```python
from build123d import *

# Parameters (mm, degrees)
SKETCH3_R           = 2.201333333
SKETCH3_R_2         = 1.693333333
BOSS_EXTRUDE1_DEPTH = 914.4
CUT_EXTRUDE1_START  = -1219.2
CUT_EXTRUDE1_DEPTH  = 1219.2


with BuildPart() as part:
    # Sketch3 → Boss-Extrude1 (new, symmetric)
    with BuildSketch(Plane.XY):
        with BuildLine():
            Line((-1.778, 0), (-1.778, 1.27))
            ThreePointArc((-1.778, 1.27), (-1.536070654, 2.494011801), (-0.846666667, 3.533942971))
            Line((-0.846666667, 3.533942971), (2.413267273, 6.793876912))
            ThreePointArc((2.413267273, 6.793876912), (2.578074335, 6.903997469), (2.772477518, 6.942666667))
            Line((2.772477518, 6.942666667), (3.048, 6.942666667))
            ThreePointArc((3.048, 6.942666667), (3.467078619, 6.769078619), (3.640666667, 6.35))
            Line((3.640666667, 6.35), (3.640666667, 4.301066667))
            ThreePointArc((3.640666667, 4.301066667), (3.948165494, 3.558698827), (4.690533333, 3.2512))
            Line((4.690533333, 3.2512), (5.300133333, 3.2512))
            ThreePointArc((5.300133333, 3.2512), (6.042501173, 3.558698827), (6.35, 4.301066667))
            Line((6.35, 4.301066667), (6.35, 10.583333333))
            ThreePointArc((6.35, 10.583333333), (5.730042687, 12.080042687), (4.233333333, 12.7))
            Line((4.233333333, 12.7), (-4.233333333, 12.7))
            ThreePointArc((-4.233333333, 12.7), (-5.730042687, 12.080042687), (-6.35, 10.583333333))
            Line((-6.35, 10.583333333), (-6.35, 0))
            Line((-6.35, 0), (-1.778, 0))
        make_face()
        with Locations(Location((-2.116666667, 8.466666667, 0), (0, 0, 180))):
            Circle(SKETCH3_R, mode=Mode.SUBTRACT)
        with Locations(Location((3.429, 9.906, 0), (0, 0, 180))):
            Circle(SKETCH3_R_2, mode=Mode.SUBTRACT)
    extrude(amount=BOSS_EXTRUDE1_DEPTH, both=True)

    # Mirror1: part across plane


with BuildPart() as part_1:
    add(part.part)
    add(part.part.mirror(Plane.ZX))

    # Sketch4 → Cut-Extrude1 (cut)
    with BuildSketch(Plane(origin=(0, 0, -914.4), x_dir=(-1, 0, 0), z_dir=(0, 0, -1)).offset(CUT_EXTRUDE1_START)):
        with BuildLine():
            Line((1.778, 1.27), (1.778, -1.27))
            ThreePointArc((1.778, -1.27), (1.536070654, -2.494011801), (0.846666667, -3.533942971))
            Line((0.846666667, -3.533942971), (-2.413267273, -6.793876912))
            ThreePointArc((-2.413267273, -6.793876912), (-2.578074335, -6.903997469), (-2.772477518, -6.942666667))
            Line((-2.772477518, -6.942666667), (-3.048, -6.942666667))
            ThreePointArc((-3.048, -6.942666667), (-3.467078619, -6.769078619), (-3.640666667, -6.35))
            Line((-3.640666667, -6.35), (-3.640666667, -4.301066667))
            ThreePointArc((-3.640666667, -4.301066667), (-3.948165494, -3.558698827), (-4.690533333, -3.2512))
            Line((-4.690533333, -3.2512), (-5.300133333, -3.2512))
            ThreePointArc((-5.300133333, -3.2512), (-6.042501173, -3.558698827), (-6.35, -4.301066667))
            Line((-6.35, -4.301066667), (-6.35, -10.583333333))
            ThreePointArc((-6.35, -10.583333333), (-5.730042687, -12.080042687), (-4.233333333, -12.7))
            Line((-4.233333333, -12.7), (4.233333333, -12.7))
            ThreePointArc((4.233333333, -12.7), (5.730042687, -12.080042687), (6.35, -10.583333333))
            Line((6.35, -10.583333333), (6.35, 10.583333333))
            ThreePointArc((6.35, 10.583333333), (5.730042687, 12.080042687), (4.233333333, 12.7))
            Line((4.233333333, 12.7), (-4.233333333, 12.7))
            ThreePointArc((-4.233333333, 12.7), (-5.730042687, 12.080042687), (-6.35, 10.583333333))
            Line((-6.35, 10.583333333), (-6.35, 4.301066667))
            ThreePointArc((-6.35, 4.301066667), (-6.042501173, 3.558698827), (-5.300133333, 3.2512))
            Line((-5.300133333, 3.2512), (-4.690533333, 3.2512))
            ThreePointArc((-4.690533333, 3.2512), (-3.948165494, 3.558698827), (-3.640666667, 4.301066667))
            Line((-3.640666667, 4.301066667), (-3.640666667, 6.35))
            ThreePointArc((-3.640666667, 6.35), (-3.467078619, 6.769078619), (-3.048, 6.942666667))
            Line((-3.048, 6.942666667), (-2.772477518, 6.942666667))
            ThreePointArc((-2.772477518, 6.942666667), (-2.578074335, 6.903997469), (-2.413267273, 6.793876912))
            Line((-2.413267273, 6.793876912), (0.846666667, 3.533942971))
            ThreePointArc((0.846666667, 3.533942971), (1.536070654, 2.494011801), (1.778, 1.27))
        make_face()
    extrude(amount=CUT_EXTRUDE1_DEPTH, mode=Mode.SUBTRACT)


solid = part_1.part
```
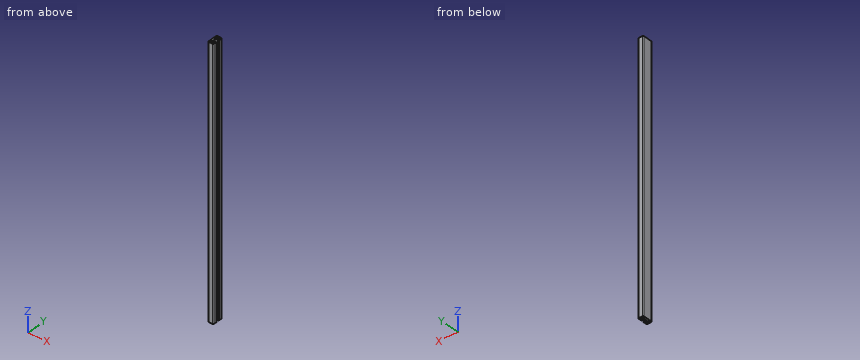
Model file for the job. Use its own axes, mm. Give positions to 0.01 mm unless a question says otherwise; leave off trailing zeros. Write each question's results on one line, items separated by ' | '.
(1) Probe line 1 along X through (y, z) = (-8.5, 502.5); line 2 along Y through (x, z) = (-0.25, 696); line 3 along Y through (x, z) = (3.5, 802). List the from-to ranges inside material, lowest first.
Geometry results:
line 1: x = -6.35 to -4.32, 0.08 to 2.49, 4.37 to 6.35 | line 2: y = -12.7 to -9.63, -7.3 to -4.13, 4.13 to 7.3, 9.63 to 12.7 | line 3: y = -12.7 to -11.6, -8.21 to -6.73, 6.73 to 8.21, 11.6 to 12.7
(2) Flat gauge pins, fed straight in: pin 1 Ø5 at (x, y) = (2.5, -5) entering from +Z; pin 2 Ø1 at (y, z) = (-1, 834) entering from +X; pin 3 Ø0.5 at (x, z) = (5, 512.5) entering from -Y. Where does each tip first touch, or does it go through?
Geometry results:
pin 1: stops at z = 914.4 | pin 2: stops at x = -1.77 | pin 3: stops at y = -12.64
(3) Cut at A-A on z = 730.5. Give the number of separate pieces and of enclosed holes in the cut face, and give its area (3 significant figures).
Geometry results:
separate pieces: 1 | enclosed holes: 4 | area: 196 mm²
